Work out the finished part from the listing and answer in its coordinate system (mm). A direction names the side the tool comes from. Give positions to 0.01 mm unless a question says otherwise; leave off trailing zeros. Order: outer loops, then holes, each group sorted by start corner. A loop starts at its lowest first (then second) coordinate and runs counter-clockwise, first axis right, second up.
Autodesk Inventor part; units mm, degrees
ref_plane "YZ Plane" through (0, 0, 0) normal (1, 0, 0) x (0, 1, 0)
ref_plane "XZ Plane" through (0, 0, 0) normal (0, 1, 0) x (-1, 0, 0)
ref_plane "XY Plane" through (0, 0, 0) normal (0, 0, 1) x (1, 0, 0)
sketch "Sketch1" plane through (0, 0, 0) normal (0, 0, 1) x (1, 0, 0)
  line L0 (0, -1.778) -> (4.6736, -1.778) construction
  line L1 (4.6736, -1.778) -> (4.6736, 4.9784) construction
  line L2 (4.6736, 4.9784) -> (0, 4.9784) construction
  line L3 (0, 4.9784) -> (0, -1.778) construction
  line L4 (0, 1.6002) -> (0, 4.0894)
  line L5 (0, 1.6002) -> (0, -0.889)
  line L6 (4.6736, 1.6002) -> (4.6736, 4.0894)
  line L7 (4.6736, 1.6002) -> (4.6736, -0.889)
  arc A0 (4.6736, 4.0894) -> (0, 4.0894) centre (2.3368, 1.4627) ccw
  arc A1 (0, -0.889) -> (4.6736, -0.889) centre (2.3368, 1.7377) ccw
  circle A2 centre (2.3368, 1.6002) radius 6.35
  dimension "d21" = 4.6736
  dimension "d22" = 6.7564
  dimension "d23" = 2.4892
  dimension "d24" = 2.4892
  dimension "d25" = 12.7
  dimension "d30" = 3.5157
  dimension "d31" = 3.5157
  dimension "d32" = 0.2751
  dimension "d33" = 2.3368
  dimension "d34" = 0.1375
  dimension "d35" = 2.3368
extrude "Extrusion1" add sketch "Sketch1" along normal blind 5.334
sketch "Sketch2" plane through (2.3876, 3.4798, 5.334) normal (0, 0, 1) x (1, 0, 0)
  circle A0 centre (0, -1.8796) radius 0.9525
  circle A1 centre (0, -1.8796) radius 12.7
  line L0 (0, 10.8204) -> (0, 4.4702) construction
  circle A2 centre (-0.0508, -1.8796) radius 6.35
  circle A3 centre (0, 7.6453) radius 0.9525
  line L1 (0, -14.5796) -> (0, -8.2294) construction
  circle A4 centre (0, -11.4045) radius 0.9525
  dimension "d26" = 1.905
  dimension "d27" = 25.4
  dimension "d28" = 1.905
  dimension "d29" = 1.905
extrude "Extrusion2" add sketch "Sketch2" along normal blind 5.08 contours A1 | A2
ref_plane "Work Plane1" through (2.3876, 3.4798, -50.8) normal (0, 0, -1) x (-1, 0, 0)
sketch "Sketch5" plane through (2.3876, 3.4798, -50.8) normal (0, 0, -1) x (-1, 0, 0)
  line L0 (2.3876, 0.6096) -> (2.3876, -4.3688)
  arc A0 (2.3876, 0.6096) -> (-2.286, 0.6096) centre (0.0508, -2.0171) ccw
  line L1 (-2.286, -4.3688) -> (-2.286, 0.6096)
  arc A1 (-2.286, -4.3688) -> (2.3876, -4.3688) centre (0.0508, -1.7421) ccw
  circle A2 centre (0.0508, -1.8796) radius 6.35
  point P0 (2.3876, -3.4798)
properties part number "Zoetrope_Motor_Connector"
1. Straight lines are drawn through the part: probe 1 along Z at (x, y) = (0.5, -6); probe 2 along Y at (x, z) = (0.75, 4.5); probe 3 along Y at (x, z) = (1.5, 0.5). For each, find the intervals that lie inside material, in ascending order.
Findings below:
probe 1: z = 5.33 to 10.41
probe 2: y = -4.55 to -1.4, 4.6 to 7.75
probe 3: y = -4.69 to -1.68, 4.88 to 7.89
2. Given P1, Ø1.4, axis at x = 3, y = 1, coming from the -Z side; P2, Ø5, axis at y = -3, z = 7, coming from the +X side; P3, Ø1.5, axis at x = 4, z = 3, coming from the +Y side; P4, Ø2, axis at x = -7.5, z = 3.5, coming from the -Y side, each flat-ended and moving along its own axis, determine where each tip first touches the part or whether it passes through.
Findings below:
P1: stops at z = 5.33
P2: stops at x = 14.91
P3: stops at y = 7.88
P4: passes through
3. Which of the six approach directions +Z, -Z, +X, -X, +Y, -Y give full straight-line access (tool end or side, diameter ignored) to faces 4 (the face through (1.686, 10.481, 7.838)), 5 (the face through (4.674, 2, 3))?
Findings below:
face 4: +Z, -Z
face 5: -Z
4. The mould has two halves that part along X. Classify faces 1 (the face through (-3.43, 4.6, 5.334)), 2 (the face through (14.501, -2.215, 7.838)), 3 (the face through (1.436, 1.558, 7.838)): pulls with the +X half, pulls with the -X half, needs draft (parallel to the pull), parting line crosses it, or undercut.
Findings below:
face 1: needs draft
face 2: parting line crosses it
face 3: undercut
5. The part is cut by section D-D (y = -4.25). Write down the section's boundary in (x, z), then the cut area to 3 significant figures.
Findings below:
outline: (-8.88, 5.33) - (-0.13, 5.33) - (-0.13, 0) - (4.81, 0) - (4.81, 5.33) - (13.66, 5.33) - (13.66, 10.41) - (-8.88, 10.41) - close
area: 141 mm2
6. The part is cut by section C-C (x = 5.5). Write down the section's boundary in (y, z).
Findings below:
outline: (-10.71, 5.33) - (-3.91, 5.33) - (-3.91, 0) - (7.11, 0) - (7.11, 5.33) - (13.91, 5.33) - (13.91, 10.41) - (-10.71, 10.41) - close
7. The part is cut by section B-B (z = 4.75). Write down the section's boundary in (x, y).
Findings below:
outline: circle Ø12.7 at (2.34, 1.6); hole (0, -0.89) arc R3.52 ccw to (4.67, -0.89) - (4.67, 4.09) arc R3.52 ccw to (0, 4.09) - close
8. The part is cut by section A-A (y = -7.5). Write down the section's boundary in (x, z), then the cut area to 3 significant figures.
Findings below:
outline: (-6.47, 5.33) - (1.54, 5.33) - (1.54, 10.41) - (-6.47, 10.41) - close; (3.24, 5.33) - (11.25, 5.33) - (11.25, 10.41) - (3.24, 10.41) - close
area: 81.3 mm2
